Can you work these out from the model? Positions are in its coordinate system, mm. A direction names the side the tool comes from. Coordinates: 2 decimals unless noted, no trailing zeros. Write each loop counter-clockwise with the first axis right and the second up, starting at its lowest first coordinate (ties: lowest second). Pieces come first, ordered by that corner, then holes.
```python
from build123d import *

# Parameters (mm, degrees)
F0_W     = 228.6
F0_H     = 38.1
F0_R     = 12.7
F1_DEPTH = 19.05
F2_W     = 136.525
F2_H     = 38.1
F2_H_2   = 53.975
F3_DEPTH = 1.5875
F4_R     = 15.875
F5_DEPTH = 50.8


with BuildPart() as f1:
    # F0 (on Top) → F1 (new body)
    with BuildSketch(Plane.XY):
        Rectangle(F0_W, F0_H)
        with Locations((-88.9, 0)):
            Circle(F0_R, mode=Mode.SUBTRACT)
        with Locations((88.9, 0)):
            Circle(F0_R, mode=Mode.SUBTRACT)
    extrude(amount=F1_DEPTH)

    # F2 (on face) → F3 (join, symmetric)
    with BuildSketch(Plane.XY.offset(19.05)):
        Rectangle(F2_W, F2_H)
        with Locations((0, 46.0375)):
            Rectangle(F2_W, F2_H_2)
        with Locations((0, -46.0375)):
            Rectangle(F2_W, F2_H_2)
    extrude(amount=F3_DEPTH, both=True)

    # F4 (on face) → F5 (join)
    with BuildSketch(Plane(origin=(0, 0, 0), x_dir=(1, 0, 0), z_dir=(0, 0, -1))):
        Circle(F4_R)
    extrude(amount=F5_DEPTH)


solid = f1.part
```
1. If I drill on L1, parallel to Y at x = -88, z = 15; L2, parallel to Z at x = 24.5, y = 63; L3, parallel to Z at x = -60, y = -4.5, over which ranges is the centre line in solid material (lowest first)?
2. If we section it at A-A, the plane y = 0: Count the separate pieces of the cut face and the enclosed holes in it, plus the area to 3 significant figures.
3. Which directions (+Z, -Z, +X, -X, +Y, -Y) give clear straight access to the entire face, cutting with the end or side of a thin tool? Please do faces 5 (the face through (-1, -46, 17.463)), 6 (the face through (101, 5, 19.05)), 7 (the face through (-102, 0, 19.05)), 8 (the face through (-1, 46, 17.463)).
4. I'm going to push flat-ended pins straight in: P1, Ø5.5, axis at x = -6.5, z = 11.5, coming from the +Y side; P2, Ø23, axis at x = 88.9, y = 0, coming from the +Z side; P3, Ø3.5, axis at y = -32.5, z = 18.5, coming from the -X side; P4, Ø5.5, axis at x = 11, z = 7.5, coming from the -Y side. Where does each tip first touch, or does it pass through?
5. We'd pull the mould along X, two halves only. Please class faces 1 (the face through (-76.786, 3.815, 9.392)), 2 (the face through (-2, -19.05, 9)), 3 (the face through (-3.441, 15.497, -25.044)), 4 (the face through (114.3, 0, 9)): released by +X, released by -X, zero draft, split by the parting line, or undercut.
6. If we section it at B-B, the plane x = 88.9: List the corners of the cut face in (y, z) for me.
7. If we section it at C-C, the plane z = 7: List the corners of the cut face in (x, y) for me, plus the area to 3 significant figures.
Answers:
1. L1: y = -19.05 to -12.67, 12.67 to 19.05
1. L2: z = 17.46 to 20.64
1. L3: z = 0 to 20.64
2. separate pieces: 3
2. enclosed holes: 0
2. area: 5,220 mm2
3. face 5: -Z, +X, -X, -Y
3. face 6: +Z, +X, +Y, -Y
3. face 7: +Z, -X, +Y, -Y
3. face 8: -Z, +X, -X, +Y
4. P1: stops at y = 19.05
4. P2: passes through
4. P3: stops at x = -68.26
4. P4: stops at y = -19.05
5. face 1: undercut
5. face 2: zero draft
5. face 3: split by the parting line
5. face 4: released by +X
6. outline: (-19.05, 0) - (-12.7, 0) - (-12.7, 19.05) - (-19.05, 19.05) - close; (12.7, 0) - (19.05, 0) - (19.05, 19.05) - (12.7, 19.05) - close
7. outline: (-114.3, -19.05) - (114.3, -19.05) - (114.3, 19.05) - (-114.3, 19.05) - close; hole circle Ø25.4 at (-88.9, 0); hole circle Ø25.4 at (88.9, 0)
7. area: 7,700 mm2
